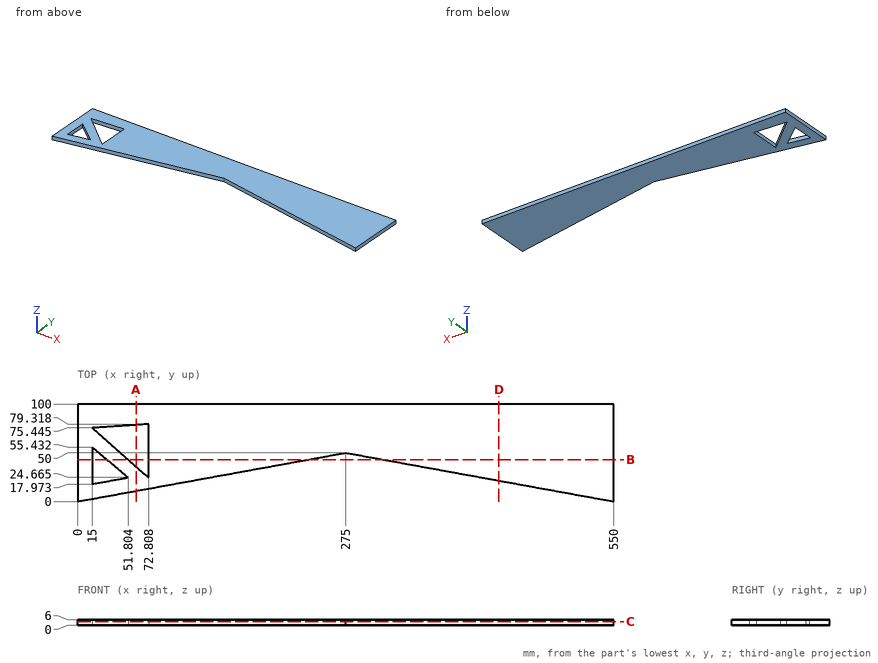
Geometry check sheet. Reference: drawing and pictorial views, mm from the part's lowest x, y, z. Round coordinates to 2 decimals unless told otherwise and drop trailing zeros. Write each loop counter-clockwise with the first axis right and the second up, starting at its lowest first coordinate (ties: lowest second). Pieces come first, ordered by that corner, then holes. Notation, with made-up numbers: (-29, 62.5) -> (-3, 62.5) arc R25 ccw to (-3, 83.5) -> close; hole circle Ø4 at (76, 13). An arc over 180 degrees is marked (long way). Put each result on its own line as item: value.
1) Cross-section at D-D, the plane x = 432. Enter the section's corners in (y, z) (1 decimal), plus the area to 3 significant figures.
Recorded:
outline: (21.5, 0) -> (100, 0) -> (100, 6) -> (21.5, 6) -> close
area: 471 mm2
2) Thickness scan on probe 1 along X at (y, z) = (54, 1.5) (1 decimal); probe 2 along X at (y, z) = (58.5, 1) (1 decimal); probe 3 along X at (y, z) = (64, 2.25) (1 decimal). Record the ranges inside material, lowest first. Write a range as from..to.
Recorded:
probe 1: x = 0..15, 16.7..39.4, 72.8..550
probe 2: x = 0..34.3, 72.8..550
probe 3: x = 0..28, 72.8..550
3) Cross-section at C-C, the plane z = 3.75. Enter the section's corners in (x, y) (1 decimal), plus the area to 3 significant figures.
Recorded:
outline: (0, 0) -> (275, 50) -> (550, 0) -> (550, 100) -> (0, 100) -> close; hole (15, 18) -> (51.8, 24.7) -> (15, 55.4) -> close; hole (15, 75.4) -> (72.8, 24.7) -> (72.8, 79.3) -> close
area: 39,000 mm2
4) Cross-section at B-B, the plane y = 43. Enter the section's corners in (x, z) (1 decimal).
Recorded:
outline: (0, 0) -> (15, 0) -> (15, 6) -> (0, 6) -> close; (29.9, 0) -> (51.9, 0) -> (51.9, 6) -> (29.9, 6) -> close; (72.8, 0) -> (236.5, 0) -> (236.5, 6) -> (72.8, 6) -> close; (313.5, 0) -> (550, 0) -> (550, 6) -> (313.5, 6) -> close
5) Cross-section at A-A, the plane x = 60. Enter the section's corners in (y, z) (1 decimal).
Recorded:
outline: (10.9, 0) -> (35.9, 0) -> (35.9, 6) -> (10.9, 6) -> close; (78.5, 0) -> (100, 0) -> (100, 6) -> (78.5, 6) -> close
